```python
from build123d import *

# Parameters (mm, degrees)
F2_DEPTH = 2.54
F3_DEPTH = 23.622
F4_SIZE  = 1.26999


# Not quite as in the source:
# - a fillet or chamfer is up to 0.001 mm smaller than in the source, because OpenCascade refuses the exact size


with BuildPart() as f2:
    # F0 (on Top) → F2 (new body)
    with BuildSketch(Plane.XY):
        Polygon((12.5471574406, 12.5223604022), (0, 46.3847853243), (-12.5471574406, 12.5223604022), (-46.1385440799, 0), (-12.5471574406, -12.5223604022), (0, -46.3847853243), (12.5471574406, -12.5223604022), (46.1385440799, 0), align=None)
    extrude(amount=F2_DEPTH)

    # F1 (on Top) → F3 (cut)
    with BuildSketch(Plane.XY):
        Polygon((5.7690664033, 5.6696828615), (0, 20.1142430305), (-5.7690664033, 5.6696828615), (-19.5389121215, -0.109308556), (-5.705270301, -5.7338749296), (0, -19.5673167638), (5.705270301, -5.7338749296), (19.5389121215, -0.109308556), align=None)
    extrude(amount=F3_DEPTH, mode=Mode.SUBTRACT)

    # F4 (size 1.27 in the source; OpenCascade refuses exactly that, so slightly less here)
    f4_edges = [f2.edges().sort_by_distance(p)[0] for p in [
        (6.273579, -29.453573, 2.54),
        (-6.273579, -29.453573, 2.54),
        (-29.342851, -6.26118, 2.54),
        (-29.342851, 6.26118, 2.54),
        (-6.273579, 29.453573, 2.54),
        (6.273579, 29.453573, 2.54),
        (29.342851, 6.26118, 2.54),
        (29.342851, -6.26118, 2.54),
        (-6.273579, 29.453573, 0),
        (29.342851, 6.26118, 0),
        (6.273579, 29.453573, 0),
        (29.342851, -6.26118, 0),
        (6.273579, -29.453573, 0),
        (-6.273579, -29.453573, 0),
        (-29.342851, -6.26118, 0),
        (-29.342851, 6.26118, 0),
        (-12.653989, 2.780187, 0),
        (12.653989, 2.780187, 2.54),
        (2.884533, 12.891963, 2.54),
        (-2.884533, 12.891963, 2.54),
        (-12.653989, 2.780187, 2.54),
        (-12.622091, -2.921592, 2.54),
        (-2.852635, -12.650596, 2.54),
        (2.852635, -12.650596, 2.54),
        (12.622091, -2.921592, 2.54),
        (-12.622091, -2.921592, 0),
        (-2.852635, -12.650596, 0),
        (2.852635, -12.650596, 0),
        (12.622091, -2.921592, 0),
        (12.653989, 2.780187, 0),
        (2.884533, 12.891963, 0),
        (-2.884533, 12.891963, 0),
    ]]
    chamfer(f4_edges, length=F4_SIZE)


solid = f2.part
```
Can you work these out from the model? Positions are in its coordinate system, mm. A direction names the side the tool comes from. Round coordinates to 2 decimals unless told otherwise and drop trailing zeros. Loops run counter-clockwise (first coordinate to the right, second up) from the corner with the lowest first, then second, coordinate; pieces in that order, holes last. Notation, with made-up numbers: (31, -9) -> (60, -9) arc R21 cw to (60, 10) -> close; hole circle Ø6 at (-31.75, -4.75). An arc over 180 degrees is marked (long way). One line per item, written item: value. Start each with the question number.
1. If we mould it in two halves opening along X, with no side actions, what happens to faces 4 (the flat face through (28.613, -5.865, 0.644)), 5 (the flat face through (14.4, -2.88, 1.9)), 6 (the flat face through (-29.091, -5.687, 0.644))? For each: pulls with the +X half, pulls with the -X half, needs draft (parallel to the pull), parting line crosses it, or undercut.
2. For pin 1 (12 mm diameter, centred on x = -13, y = 33, fed in from -Z), with a flat end and sliding along its axis, tell me the tip position at first contact or that it passes through.
3. If I drill on probe 1 along Y at (x, z) = (19.5, 2); probe 2 along X at (y, z) = (14, 1.45); probe 3 along Y at (x, z) = (-14.5, 1), over which ranges is the centre line in solid material (lowest first)?
4. For faces 1 (the flat face through (-29.091, -5.687, 1.896)), 2 (the flat face through (2.8, -14.43, 0.64)), 3 (the flat face through (2.893, -14.196, 1.896)), which set-ups out of +Z, -Z, +X, -X, +Y, -Y let a thin tool reach every point of the face, with its end or its side?
5. If we section it at C-C, the plane z = 0.8: Write out the boundary of the cut face in (x, y), then the cut area to 3 significant figures.
Calculated:
1. face 4: pulls with the +X half
1. face 5: undercut
1. face 6: pulls with the -X half
2. pin 1: passes through
3. probe 1: y = -9.15 to -0.91, 0.7 to 9.15
3. probe 2: x = -11.81 to -2.64, 2.64 to 11.81
3. probe 3: y = -11.51 to -2.45, 2.3 to 11.51
4. face 1: +Z, -X, -Y
4. face 2: -Z
4. face 3: +Z
5. outline: (-44.79, 0) -> (-12.18, -12.16) -> (0, -45.03) -> (12.18, -12.16) -> (44.79, 0) -> (12.18, 12.16) -> (0, 45.03) -> (-12.18, 12.16) -> close; hole (-20.77, -0.12) -> (-6.06, -6.1) -> (0, -20.8) -> (6.06, -6.1) -> (20.77, -0.12) -> (6.13, 6.03) -> (0, 21.38) -> (-6.13, 6.03) -> close
5. area: 1,680 mm²
